The listing builds one solid part. Answer for the finished solid, in the listing's coordinates (mm). Face numbers are marked on the shaded views. Round coordinates to 2 decimals unless told otherwise and drop trailing zeros. Loops run counter-clockwise (first coordinate to the right, second up) from the corner with the lowest first, then second, coordinate; pieces in that order, holes last. Notation, with made-up numbers: (5, 84.25) - (20, 84.25) arc R21 cw to (20, 119.25) - close; hole circle Ø7 at (61.5, 83). An arc over 180 degrees is marked (long way). One line per item, written item: value.
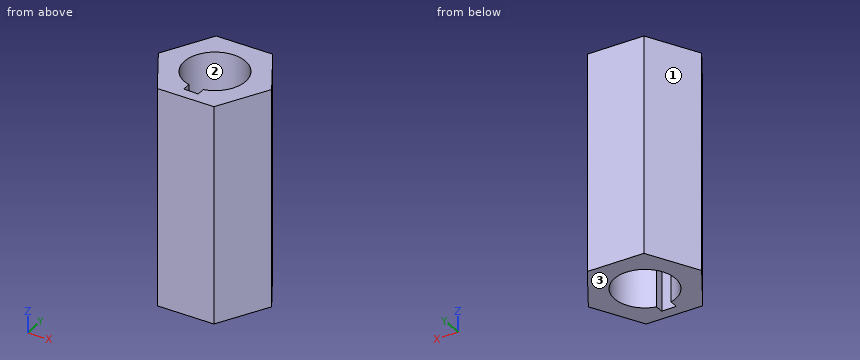
```python
from build123d import *

# Parameters (mm, degrees)
SKETCH1_R           = 4
BOSS_EXTRUDE1_DEPTH = 28.575
SKETCH2_W           = 1.905
SKETCH2_H           = 1.905
CUT_EXTRUDE1_DEPTH  = 29.575


with BuildPart() as part:
    # Sketch1 → Boss-Extrude1 (new body)
    with BuildSketch(Plane.XY):
        Polygon((-7.329405666, -0.20771595), (-3.484815544, -6.451309476), (3.844590123, -6.243593526), (7.329405666, 0.20771595), (3.484815544, 6.451309476), (-3.844590123, 6.243593526), align=None)
        Circle(SKETCH1_R, mode=Mode.SUBTRACT)
    extrude(amount=BOSS_EXTRUDE1_DEPTH)

    # Sketch2 → Cut-Extrude1 (cut, through all)
    with BuildSketch(Plane.XY.offset(28.575)):
        with Locations((0, -4)):
            Rectangle(SKETCH2_W, SKETCH2_H)
    extrude(amount=-CUT_EXTRUDE1_DEPTH, mode=Mode.SUBTRACT)


solid = part.part
```
1) Consider L1, parallel to Y at x = -2.25, z = 19.25; L2, parallel to Y at x = -1, z = 12.5; L3, parallel to X at y = -4.25, z = 27.25. Determine where each line is inside the solid, lowest interval first.
Final values:
L1: -6.42 to -3.31, 3.31 to 6.29
L2: -6.38 to -3.87, 3.87 to 6.32
L3: -4.84 to -0.95, 0.95 to 4.92
2) A cutting plane is placed at A-A on z = 13.25. Give the vertices of the cut face in (x, y), and give its area (3 significant figures).
Final values:
outline: (-7.33, -0.21) - (-3.48, -6.45) - (3.84, -6.24) - (7.33, 0.21) - (3.48, 6.45) - (-3.84, 6.24) - close; hole (-0.95, -4.95) - (0.95, -4.95) - (0.95, -3.88) arc R4 ccw (long way) to (-0.95, -3.88) - close
area: 87.5 mm2
3) A cutting plane is placed at D-D on x = 4.5. Give the vertices of the cut face in (y, z) (3 decimals).
Final values:
outline: (-5.03, 0) - (4.803, 0) - (4.803, 28.575) - (-5.03, 28.575) - close
4) A cutting plane is placed at B-B on y = -2.75. Give the vertices of the cut face in (x, z) (3 decimals).
Final values:
outline: (-5.764, 0) - (-2.905, 0) - (-2.905, 28.575) - (-5.764, 28.575) - close; (2.905, 0) - (5.732, 0) - (5.732, 28.575) - (2.905, 28.575) - close
5) A cutting plane is placed at C-C on x = 0. Give the vertices of the cut face in (y, z) (1 decimal).
Final values:
outline: (-6.4, 0) - (-5, 0) - (-5, 28.6) - (-6.4, 28.6) - close; (4, 0) - (6.4, 0) - (6.4, 28.6) - (4, 28.6) - close
6) For a pull along X with two mould halves and no side action, classify the marked faces 1, 2 and 3 as released by +X, released by -X, zero draft, split by the parting line, or undercut.
Final values:
face 1: released by -X
face 2: undercut
face 3: zero draft
7) Each of these flat-tipped pins is pushed along its axis until it touches: pin 1 Ø6 at (y, z) = (3, 11) entering from +X; pin 2 Ø1.2 at (y, z) = (-4.5, 12.5) entering from -X; pin 3 Ø2 at (x, z) = (0, 18) entering from +Y; pin 4 Ø1 at (x, z) = (3.5, 12) entering from -Y. Where does it stop, or does it pass through?
Final values:
pin 1: x = 7.33
pin 2: x = -5.06
pin 3: y = 6.38
pin 4: y = -6.27
